Geometry: final body of the model. Coordinates: model frame, mm. A direction names the side the tool comes from. Round coordinates to 2 decimals unless told otherwise and drop trailing zeros. Order: outer loops, then holes, each group sorted by start corner. A loop starts at its lowest first (then second) coordinate and runs counter-clockwise, first axis right, second up. Notation, with made-up numbers: (45.5, 28.25) -> (63.5, 28.25) arc R30 ccw to (63.5, 58.25) -> close; hole circle Ø3 at (-24.75, -1.75). An arc over 180 degrees is marked (long way). Put each result on its own line as item: value.
```python
from build123d import *

# Parameters (mm, degrees)
PAD_DEPTH = 4
FILLET_R  = 0.5


with BuildPart() as part:
    # Sketch → Pad (new body)
    with BuildSketch(Plane.XY):
        Polygon((-2.32, 0), (2.32, 0), (2.32, 1.64), (1.5, 1.64), (1.5, 3.32), (4, 3.32), (4, -1.68), (-4, -1.68), (-4, 3.32), (-1.5, 3.32), (-1.5, 1.64), (-2.32, 1.64), align=None)
    extrude(amount=PAD_DEPTH)

    # Fillet
    fillet_edges = [part.edges().sort_by_distance(p)[0] for p in [
        (2.32, 0.82, 4),
        (-2.32, 0.82, 4),
        (2.32, 0.82, 0),
        (-2.32, 0.82, 0),
    ]]
    fillet(fillet_edges, radius=FILLET_R)


solid = part.part
```
1. Material intervals for probe 1 along X at (y, z) = (0.9, 2.5); probe 2 along X at (y, z) = (1.7, 2.85); probe 3 along Y at (x, z) = (1.75, 3), sorted ascending.
Ans:
probe 1: -4 to -2.32, 2.32 to 4
probe 2: -4 to -1.5, 1.5 to 4
probe 3: -1.68 to 0, 1.64 to 3.32
2. Cut plane B-B on y = 2.6. Return loops of the section in (x, z), and give its area (3 significant figures).
Ans:
outline: (-4, 0) -> (-1.5, 0) -> (-1.5, 4) -> (-4, 4) -> close; (1.5, 0) -> (4, 0) -> (4, 4) -> (1.5, 4) -> close
area: 20.0 mm²
3. Draft query along X for faces 1 (the face through (-4, 1, 2)), 2 (the face through (-1.5, 2, 2)), 3 (the face through (0, -1.68, 2)). Return one class per face: +X half, -X half, draft (parallel to the pull), parting line (faces both ways), or undercut.
Ans:
face 1: -X half
face 2: undercut
face 3: draft
4. Cut plane A-A on x = 2. Return loops of the section in (y, z), and give its area (3 significant figures).
Ans:
outline: (-1.68, 0) -> (0, 0) -> (0, 4) -> (-1.68, 4) -> close; (1.64, 0) -> (3.32, 0) -> (3.32, 4) -> (1.64, 4) -> close
area: 13.4 mm²
5. Contact query for a flat-ended pin moving along its axis: P1, Ø3, axis at x = 0.5, y = 2, coming from the -Z side. Output: stop coordinate, or through.
Ans:
P1: z = 0
6. Set-up query: faces 4 (the face through (0.1, -0.3, 0)), 5 (the face through (1.5, 2, 2)), 6 (the face through (2.32, 1, 2)). Return all of +Z, -Z, +X, -X, +Y, -Y with unobstructed straight access to the full face (end or side cutting, diameter ignored); none if empty.
Ans:
face 4: -Z, +X, -X, +Y, -Y
face 5: +Z, -Z, +Y
face 6: +Z, -Z
7. Cut plane C-C on z = 1.9. Return loops of the section in (x, y), and give its area (3 significant figures).
Ans:
outline: (-4, -1.68) -> (4, -1.68) -> (4, 3.32) -> (1.5, 3.32) -> (1.5, 1.64) -> (2.32, 1.64) -> (2.32, 0) -> (-2.32, 0) -> (-2.32, 1.64) -> (-1.5, 1.64) -> (-1.5, 3.32) -> (-4, 3.32) -> close
area: 27.4 mm²
8. Cut plane D-D on y = 0.45. Return loops of the section in (x, z), and give its area (3 significant figures).
Ans:
outline: (-4, 0) -> (-2.82, 0) arc R0.5 ccw to (-2.32, 0.5) -> (-2.32, 3.5) arc R0.5 ccw to (-2.82, 4) -> (-4, 4) -> close; (2.32, 0.5) arc R0.5 ccw to (2.82, 0) -> (4, 0) -> (4, 4) -> (2.82, 4) arc R0.5 ccw to (2.32, 3.5) -> close
area: 13.2 mm²
